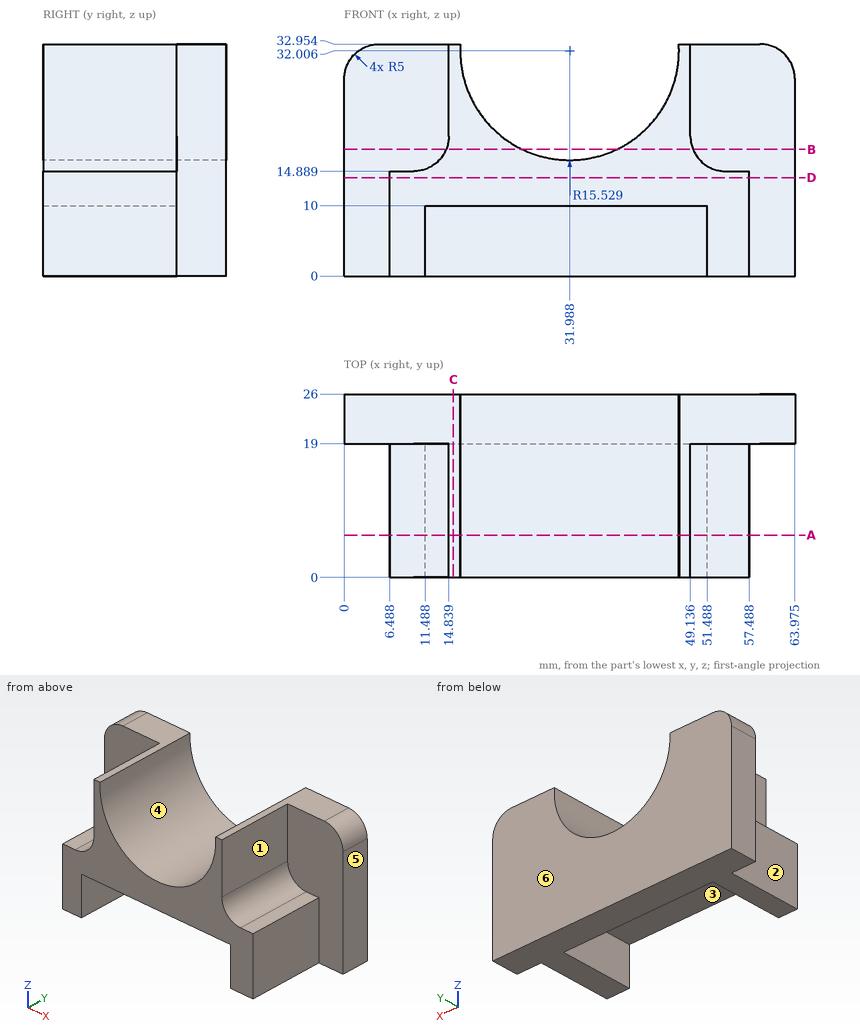
Part print with two shaded views. Sizes in mm from the minimum x, y, z corner. A direction names the side the tool comes from. Give positions to 0.01 mm unless a question says otherwise; leave off trailing zeros. Order: outer loops, then holes, each group sorted by start corner. A loop starts at its lowest first (then second) coordinate and runs counter-clockwise, first axis right, second up.
1) Saw through at D-D, the plane z = 14. Write the cut outline in (x, y) (1 decimal).
2) Pin check, flat tips, straight feed: pin 1 (16.5 mm diameter, centred on x = 5.5, z = 12, fed in from -Y); pin 2 (14.5 mm diameter, centred on y = 8, z = 23.5, fed in from -X); pin 3 (4.5 mm diameter, centred on y = 9, z = 6.5, fed in from +X); pin 4 (2 mm diameter, centred on x = 38.5, y = 4, fed in from -Z). Stop position of each tip, or through.
3) 3-axis set-ups, long thin cutter, end or side, ignore diameter. For the marked faces 1, 2 and 3: which of +Z, -Z, +X, -X, +Y, -Y reach the whole face in a straight line?
4) Wall check: probe 1 along Y at (x, z) = (19, 5.5); probe 2 along X at (y, z) = (16, 8); probe 3 along X at (y, z) = (6.75, 28.5) (1 decimal). Give the ranges that are in metal, low to high.
5) Saw through at A-A, the plane y = 6. Write the cut outline in (x, z).
6) Saw through at C-C, the plane x = 15.5. Write the cut outline in (y, z).
7) Mould opens along X. For the marked faces 4, 5 and 6 say: +X half, -X half, draft (parallel to the pull), parting line (faces both ways), or undercut.
8) Saw through at B-B, the plane z = 18. Write the cut outline in (x, y) (1 decimal).
Computed:
1. outline: (0, 19) - (6.5, 19) - (6.5, 0) - (57.5, 0) - (57.5, 19) - (64, 19) - (64, 26) - (0, 26) - close
2. pin 1: stops at y = 0
2. pin 2: stops at x = 13.27
2. pin 3: stops at x = 57.49
2. pin 4: stops at z = 10
3. face 1: +Z, +X, -Y
3. face 2: +Z, -Z, -X, -Y
3. face 3: -Z, -Y
4. probe 1: y = 19 to 26
4. probe 2: x = 6.49 to 11.49, 51.49 to 57.49
4. probe 3: x = 14.8 to 16.9, 47.1 to 49.1
5. outline: (6.49, 0) - (11.49, 0) - (11.49, 10) - (51.49, 10) - (51.49, 0) - (57.49, 0) - (57.49, 14.89) - (54.14, 14.89) arc R5 cw to (49.14, 19.89) - (49.14, 32.95) - (47.49, 32.95) arc R15.53 cw (long way) to (16.49, 32.95) - (14.84, 32.95) - (14.84, 19.89) arc R5 cw to (9.84, 14.89) - (6.49, 14.89) - close
6. outline: (0, 10) - (19, 10) - (19, 0) - (26, 0) - (26, 32.95) - (0, 32.95) - close
7. face 4: undercut
7. face 5: +X half
7. face 6: draft
8. outline: (0, 19) - (14.5, 19) - (14.5, 0) - (25.3, 0) - (25.3, 26) - (0, 26) - close; (38.7, 0) - (49.5, 0) - (49.5, 19) - (64, 19) - (64, 26) - (38.7, 26) - close
